Autodesk Inventor part; units mm, degrees
ref_plane "YZ Plane" through (0, 0, 0) normal (1, 0, 0) x (0, 1, 0)
ref_plane "XZ Plane" through (0, 0, 0) normal (0, 1, 0) x (-1, 0, 0)
ref_plane "XY Plane" through (0, 0, 0) normal (0, 0, 1) x (1, 0, 0)
sketch "スケッチ1" plane through (0, 0, 0) normal (0, 1, 0) x (-1, 0, 0)
  line L0 (101.7324, -28.9004) -> (451.7324, -28.9004)
  line L1 (451.7324, -28.9004) -> (451.7324, 67.6956)
  arc A0 (451.7324, 67.6956) -> (328.1926, 37.3714) centre (451.7324, -199.1148) ccw
  arc A1 (101.7324, -28.9004) -> (328.1926, 37.3714) centre (48.6916, 572.4068) ccw
  dimension "d1" = 350
  dimension "d2" = 603.642
extrude "押し出し1" add sketch "スケッチ1" along normal blind 70
sketch "スケッチ2" plane through (-101.7324, 0, -28.9004) normal (0, 0, -1) x (-1, 0, 0)
  arc A0 (68.7528, 0) -> (350, 70) centre (68.7528, 600) ccw
  line L0 (350, 0) -> (0, 0)
  line L1 (350, 0) -> (350, 70)
  line L2 (0, 0) -> (0, 70)
  point P0 (-101.7324, 0)
  dimension "d9" = 600
extrude "押し出し2" cut sketch "スケッチ2" against normal through all
shell "シェル1" thickness 2 removed faces 4 at (-334.0598, 39.1147, 40.3449) at (-150.6861, 46.6667, -22.5561) at (-359.2071, 70, 10.3289) at (-325.356, 65.1801, -28.9004)
sketch "スケッチ5" plane through (0, 0, 0) normal (0, 1, 0) x (-1, 0, 0)
  arc A0 (101.7324, -28.9004) -> (170.4851, -18.8207) centre (48.6916, 572.4068) ccw
  spline S0 degree 7 poles (328.1926, 37.3714) (308.4164, 27.0404) (287.5942, 17.2484) (265.7943, 8.15) (243.0935, -0.1185) (219.5774, -7.4369) (195.3405, -13.7005) (170.4851, -18.8207) knots 0 0 0 0 0 0 0 0 1 1 1 1 1 1 1 1
  arc A1 (101.7324, -28.9004) -> (170.4851, -18.8207) centre (48.6916, 572.4068) ccw
  arc A2 (170.4851, -18.8207) -> (328.1926, 37.3714) centre (48.6916, 572.4068) ccw
  arc A3 (101.5566, -26.9081) -> (205.5189, -8.436) centre (48.6916, 572.4068) ccw
  arc A4 (205.5189, -8.436) -> (327.2665, 39.1441) centre (48.6916, 572.4068) ccw
  arc A5 (101.7324, -28.9004) -> (170.4851, -18.8207) centre (48.6916, 572.4068) ccw
  line L0 (101.5566, -26.9081) -> (101.7324, -28.9004)
  line L1 (327.2665, 39.1441) -> (328.1926, 37.3714)
  point P0 (0, 0)
  dimension "d11" = 2
extrude "押し出し3" add sketch "スケッチ5" along normal blind 35 and the other way blind 10
properties part number "splitter"
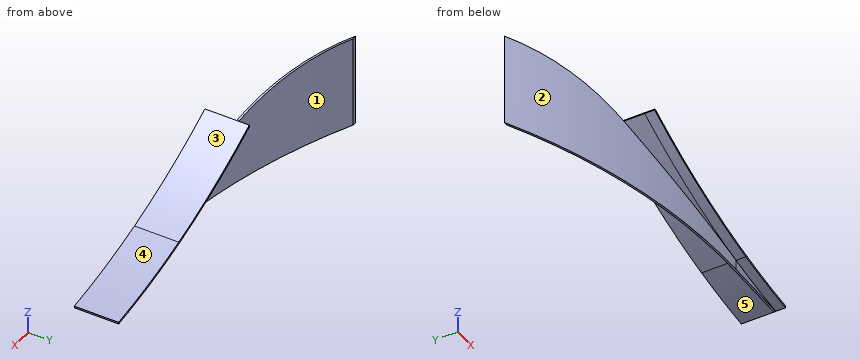
Can you work these out from the model? Positions are in its coordinate system, mm. Face numbers are marked on the shaded views. A direction names the side the tool comes from. Round coordinates to 2 decimals unless told otherwise and drop trailing zeros. Loops run counter-clockwise (first coordinate to the right, second up) from the corner with the lowest first, then second, coordinate; pieces in that order, holes last.
Item 1: If we mould it in two halves opening along Z, with no side actions, what happens to the marked faces 4 and 5? For each: +Z half, -Z half, draft (parallel to the pull), parting line (faces both ways), or undercut.
Item 2: Please list where these lines run through material, in increasing order: L1, parallel to X at y = 66.5, z = 31.5; L2, parallel to X at y = 63, z = 50; L3, parallel to Y at x = -420, z = 57.5.
Item 3: Suppose I cut it at C-C, the plane z = 62.5. Write out the boundary of the cut face in (x, y).
Item 4: Which directions (+Z, -Z, +X, -X, +Y, -Y) give clear straight access to the entire face, cutting with the end or side of a thin tool? Please do the marked faces 1, 2 and 3.
Item 5: Will these pins go through, and if not, where does the flat tip stop? pin 1 Ø1.5 at (x, y) = (-159, 4) entering from +Z; pin 2 Ø1.5 at (y, z) = (61, 54.5) entering from -X; pin 3 Ø6 at (y, z) = (0, 39) entering from -X.
Item 6: Suppose I cut it at B-B, the plane y = 49. Write out the boundary of the cut face in (x, z).
Reported:
1. face 4: +Z half
1. face 5: -Z half
2. L1: x = -445.04 to -440.64
2. L2: x = -438.12 to -433.61
2. L3: y = 54.34 to 56.54
3. outline: (-451.73, 70) arc R600 ccw to (-399.34, 45.36) - (-399.34, 47.52) arc R598 cw to (-447.44, 70) - close
4. face 1: -Z, +Y
4. face 2: -Z, -X, -Y
4. face 3: +Z, +X, +Y, -Y
5. pin 1: stops at z = -18.9
5. pin 2: stops at x = -435.6
5. pin 3: stops at x = -328.19
6. outline: (-407.97, -28.9) - (-402.87, -28.9) - (-402.87, 63.18) arc R266.81 ccw to (-407.97, 64.08) - close
